Autodesk Inventor part; units mm, degrees
ref_plane "YZ Plane" through (0, 0, 0) normal (1, 0, 0) x (0, 1, 0)
ref_plane "XZ Plane" through (0, 0, 0) normal (0, 1, 0) x (-1, 0, 0)
ref_plane "XY Plane" through (0, 0, 0) normal (0, 0, 1) x (1, 0, 0)
sketch "Sketch1" plane through (0, 0, 0) normal (0, 0, 1) x (1, 0, 0)
  arc A0 (28.3106, 6.35) -> (-28.3106, 6.35) centre (0, 0) ccw construction
  arc A1 (31.1988, 6.9978) -> (-31.1988, 6.9978) centre (0, 0) ccw
  arc A2 (25.4224, 5.7022) -> (-25.4224, 5.7022) centre (0, 0) ccw
  arc A3 (25.4224, 5.7022) -> (31.1988, 6.9978) centre (28.3106, 6.35) ccw
  arc A4 (-31.1988, 6.9978) -> (-25.4224, 5.7022) centre (-28.3106, 6.35) ccw
  dimension "d0" = 2.96
  dimension "d1" = 26.054
  dimension "d2" = 6.35
  dimension "d5" = 31.974
extrude "Extrusion1" add sketch "Sketch1" along normal blind 12.7
sketch "Sketch2" plane through (0, 0, 0) normal (0, 0, -1) x (-1, 0, 0)
  arc A0 (31.1988, 6.9978) -> (-31.1988, 6.9978) centre (0, 0) ccw
  arc A1 (44.3474, 11.1189) -> (-44.4956, 10.5098) centre (0, 0) ccw
  arc A2 (-44.4956, 10.5098) -> (-42.3638, 6.9657) centre (-41.6149, 9.8294) ccw
  line L0 (-42.3638, 6.9657) -> (-29.0595, 3.4863)
  arc A3 (-31.1988, 6.9978) -> (-25.4224, 5.7022) centre (-28.3106, 6.35) ccw
  arc A4 (25.4224, 5.7022) -> (31.1988, 6.9978) centre (28.3106, 6.35) ccw
  line L1 (29.1807, 3.5208) -> (42.3463, 7.5698)
  arc A5 (42.3463, 7.5698) -> (44.3474, 11.1189) centre (41.4762, 10.3991) ccw
  arc A6 (-31.1988, 6.9978) -> (-25.4224, 5.7022) centre (-28.3106, 6.35) ccw
  dimension "d6" = 45.72
extrude "Extrusion2" add sketch "Sketch2" against normal blind 3.175
sketch "Sketch3" plane through (0, 0, 3.175) normal (0, 0, 1) x (1, 0, 0)
  circle A0 centre (-26.9408, 26.9408) radius 2.667
  line L0 (0, 0) -> (0, 4.8755)
  circle A1 centre (0, 38.1) radius 2.667
  circle A2 centre (26.9408, 26.9408) radius 2.667
  dimension "d9" = 5.334
  dimension "d10" = 38.1
  dimension "d11" = 45
  dimension "d14" = 90
extrude "Extrusion3" cut sketch "Sketch3" against normal through all
properties part number "HoseClampShaftCollarShooterMount"
Design review of the part built by this model. Coordinates are the model's own, in mm. A direction names the side the tool comes from. Round coordinates to 2 decimals unless told otherwise and drop trailing zeros. Order: outer loops, then holes, each group sorted by start corner. A loop starts at its lowest first (then second) coordinate and runs counter-clockwise, first axis right, second up. Notation, with made-up numbers: M 70.5,76 L 112.5,76 A16 cw 112.5,102 Z; hole C -36.75,-31 d11. An arc over 180 degrees is marked long. Put each result on its own line as item: value.
Q1. Consider section C-C (x = -15). State the section outline as (y, z) points (3 decimals).
Reported:
outline: M 21.303,0 L 43.189,0 L 43.189,3.175 L 28.237,3.175 L 28.237,12.7 L 21.303,12.7 Z
Q2. Machinability: for faces 1 (the face through (-0.15, 26.22, 12.7)), 2 (the face through (-0.6, 31.97, 7.87)), which of the approach directions +Z, -Z, +X, -X, +Y, -Y give a long, thin tool a straight path to every point of the face, cutting with its end or side? Answer none if there is none.
Reported:
face 1: +Z, +X, -X, +Y, -Y
face 2: +Z, +Y
Q3. Insertion check: pin 1 Ø1.5 at (x, y) = (-32, 27) entering from +Z (3 decimals); pin 2 Ø2 at (x, z) = (6.5, 10.5) entering from -Y; pin 3 Ø2 at (y, z) = (23.5, 5) entering from -X. Each pin has a flat end and moves straight along its axis. Give the tip position at first contact, or say it passes through.
Reported:
pin 1: z = 3.175
pin 2: y = 24.95
pin 3: x = -22.72
Q4. Draft analysis for pull direction Y (two halves, no side actions). For faces 3 (the face through (29.404, 25.919, 1.61)), 4 (the face through (-0.539, 45.717, 1.565)), 5 (the face through (44.168, 8.331, 1.565)), state which applies: released by +Y, released by -Y, zero draft, split by the parting line, or undercut.
Reported:
face 3: undercut
face 4: released by +Y
face 5: split by the parting line
Q5. Consider section D-D (z = 5.75). State the section outline as (x, y) points, and give its area (3 significant figures).
Reported:
outline: M -31.2,7 A2.96 ccw -25.42,5.7 A26.05 cw 25.42,5.7 A2.96 ccw 31.2,7 A31.97 ccw Z
area: 491 mm²
Q6. Consider section B-B (y = 38.1). State the section outline as (x, z) points (3 decimals), and give its area (3 significant figures).
Reported:
outline: M -25.273,0 L -2.667,0 L -2.667,3.175 L -25.273,3.175 Z; M 2.667,0 L 25.273,0 L 25.273,3.175 L 2.667,3.175 Z
area: 144 mm²
Q7. To check wall thickness, follow line 1 (Y direction, x = 0, z = 1.9); line 2 (X direction, y = 14, z = 2.5); line 3 (Y direction, x = -29, z = 0.5). State the ranges of each line that lie inside material, in increasing order.
Reported:
line 1: 26.05 to 35.43, 40.77 to 45.72
line 2: -43.52 to -21.97, 21.97 to 43.52
line 3: 3.47 to 25.25, 28.64 to 35.35
Q8. Consider section A-A (x = 0). State the section outline as (y, z) points (3 decimals).
Reported:
outline: M 26.054,0 L 35.433,0 L 35.433,3.175 L 31.974,3.175 L 31.974,12.7 L 26.054,12.7 Z; M 40.767,0 L 45.72,0 L 45.72,3.175 L 40.767,3.175 Z
